Geometry check sheet. Reference: the model listing, model coordinates, mm. A direction names the side the tool comes from. Coordinates: 2 decimals unless noted, no trailing zeros. Order: outer loops, then holes, each group sorted by start corner. A loop starts at its lowest first (then second) coordinate and runs counter-clockwise, first axis right, second up. Notation, with made-up numbers: (-12, 75.5) - (22, 75.5) arc R14 cw to (22, 93.5) - close; hole circle Ø1 at (16.5, 25). An arc over 180 degrees is marked (long way). Put each result on its own line as item: value.
from build123d import *

# Parameters (mm, degrees)
SKETCH1_W           = 10
SKETCH1_H           = 2
BOSS_EXTRUDE1_DEPTH = 50
FILLET1_R           = 2
FILLET2_R           = 4
FILLET3_R           = 2


with BuildPart() as part:
    # Sketch1 → Boss-Extrude1 (new body)
    with BuildSketch(Plane(origin=(0, 0, 0), x_dir=(1, 0, 0), z_dir=(0, 1, 0))):
        Polygon((3, 4.05), (0, 4.05), (0, -4.05), (8, -4.05), (8, 4.05), align=None)
        Polygon((3, 11.05), (3, 4.05), (8, 4.05), (8, 9.05), (8, 11.05), align=None)
        Polygon((-2.04, 7.95), (0, 7.95), (0, -7.95), (-2.04, -7.95), (-6.152414984, -4.048), (-6.152414984, 4.048), align=None)
        with Locations((13, 10.05)):
            Rectangle(SKETCH1_W, SKETCH1_H)
    extrude(amount=BOSS_EXTRUDE1_DEPTH)

    # Fillet1
    fillet1_edges = [part.edges().sort_by_distance(p)[0] for p in [
        (8, 25, -9.05),
    ]]
    fillet(fillet1_edges, radius=FILLET1_R)

    # Fillet2
    fillet2_edges = [part.edges().sort_by_distance(p)[0] for p in [
        (8, 25, 4.05),
    ]]
    fillet(fillet2_edges, radius=FILLET2_R)

    # Fillet3
    fillet3_edges = [part.edges().sort_by_distance(p)[0] for p in [
        (18, 25, -9.05),
    ]]
    fillet(fillet3_edges, radius=FILLET3_R - 0.0001)  # a hair under: the kernel refuses the full size


solid = part.part
Q1. Access from +Z, -Z, +X, -X, +Y, -Y to the whole of each face (thin tool, end or side, straight path). Record for faces 1 (the flat face through (3, 25, -8)), 2 (the flat face through (-1, 25, -7.95)), 3 (the flat face through (13, 25, -9.05)).
Answer block:
face 1: -Z, +Y, -Y
face 2: -Z, -X, +Y, -Y
face 3: +Z, +X, +Y, -Y
Q2. Section check B-B on x = 2.5. Record the boundary of the cut face in (y, z).
Answer block:
outline: (0, -4.05) - (50, -4.05) - (50, 4.05) - (0, 4.05) - close
Q3. Depth check by flat-ended pin: pin 1 Ø5 at (y, z) = (38, -7.5) entering from +X; pin 2 Ø5 at (x, y) = (3.5, 17.5) entering from +Z; pin 3 Ø1.5 at (y, z) = (38.5, -7) entering from +X. Enter the tip coordinate at first touch or a pass-through.
Answer block:
pin 1: stops at x = 17.7
pin 2: stops at z = 4.05
pin 3: stops at x = 8.13
Q4. Thickness scan on L1, parallel to Z at x = 10.75, y = 25; L2, parallel to X at y = 20, z = -4; L3, parallel to Z at x = -1, y = 29. Record the ranges inside material, lowest first. Write a range as [from, to].
Answer block:
L1: z = [-11.05, -9.05]
L2: x = [-6.15, 8]
L3: z = [-7.95, 7.95]
Q5. Section check C-C on z = -0.5. Record the boundary of the cut face in (x, y), then the cut area to 3 significant figures.
Answer block:
outline: (-6.15, 0) - (8, 0) - (8, 50) - (-6.15, 50) - close
area: 708 mm^2
Q6. Draft check along X on faces 4 (the cylindrical face through (8.57, 25.35, -8.45)), 5 (the flat face through (3, 0, -2)), 6 (the flat face through (2, 25, -4.05)). Enter one of: pulls with the +X half, pulls with the -X half, needs draft (parallel to the pull), parting line crosses it, or undercut.
Answer block:
face 4: pulls with the +X half
face 5: needs draft
face 6: undercut
